Check sheet for the drawn part. Datum: minimum x, y, z corner. Units: mm. A direction names the side the tool comes from. Round coordinates to 2 decimals unless told otherwise and drop trailing zeros. Order: outer loops, then holes, each group sorted by start corner. A loop starts at its lowest first (then second) coordinate and runs counter-clockwise, first axis right, second up. Notation, with made-up numbers: (21, 32.5) -> (46, 32.5) arc R12 cw to (46, 53.5) -> close; hole circle Ø9 at (88, 28). An arc over 180 degrees is marked (long way). Answer as a JSON object with one key per item and string values. Group by question number.
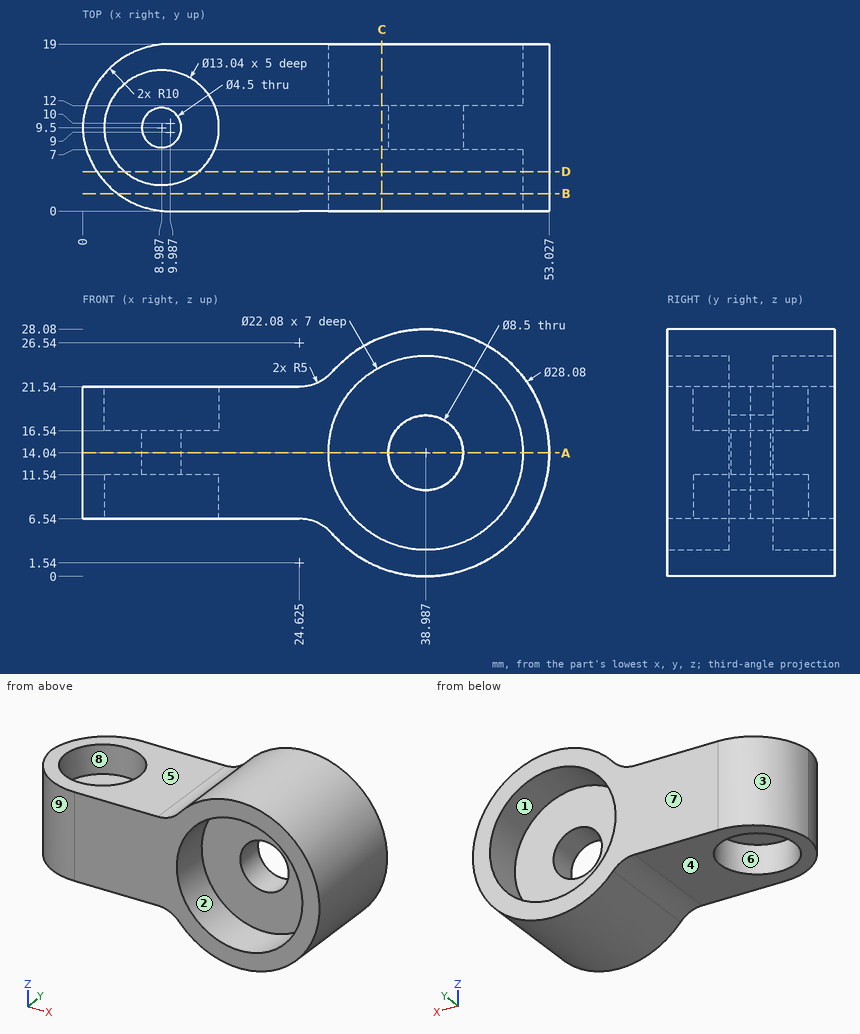
Item 1: Sectioned sample at A-A, the plane z = 14.04. Enter the section's corners in (x, y), then the cut area to 3 significant figures.
Item 2: Thickness scan on L1, parallel to X at y = 8.3, z = 14.04 (1 decimal); L2, parallel to X at y = 15.5, z = 20 (1 decimal); L3, parallel to Y at x = 29, z = 18.25. Record the ranges inside material, lowest first.
Item 3: Mould release check, pull along Y, two halves, no side actions. Record for the marked faces 6, 7, 8 and 9: pulls with the +Y half, pulls with the -Y half, needs draft (parallel to the pull), parting line crosses it, or undercut.
Item 4: Sectioned sample at D-D, the plane y = 4.5. Enter the section's corners in (x, z) (1 decimal).
Item 5: Set-up check for the marked faces 1, 2, 3, 4 and 5: record each of +Z, -Z, +X, -X, +Y, -Y from which the full face is reachable in a straight line by a thin tool's end or side.
Item 6: Depth check by flat-ended pin: pin 1 Ø8 at (x, y) = (21.5, 3) entering from -Z; pin 2 Ø5 at (x, y) = (8.99, 9.5) entering from +Z; pin 3 Ø5.5 at (x, y) = (13.5, 11.5) entering from +Z. Enter the tip coordinate at first touch or a pass-through.
Item 7: Sectioned sample at B-B, the plane y = 2. Enter the section's corners in (x, z) (1 decimal), then the cut area to 3 significant figures.
Item 8: Sectioned sample at C-C, the plane x = 34. Enter the section's corners in (y, z) (1 decimal).
Result:
{
 "1": {"outline": "(0, 9.5) arc R10 ccw to (9.99, 0) -> (27.95, 0) -> (27.95, 7) -> (34.74, 7) -> (34.74, 12) -> (27.95, 12) -> (27.95, 19) -> (9.99, 19) arc R10 ccw to start; (43.24, 7) -> (50.03, 7) -> (50.03, 0) -> (53.03, 0) -> (53.03, 19) -> (50.03, 19) -> (50.03, 12) -> (43.24, 12) -> close; hole circle Ø4.5 at (8.99, 9.5)", "area": "597 mm2"},
 "2": {"L1": "x = 0.1 to 7.1, 10.9 to 34.7, 43.2 to 53", "L2": "x = 2.4 to 6.4, 11.5 to 29.7, 48.3 to 51.7", "L3": "y = 7 to 12"},
 "3": {"face 6": "undercut", "face 7": "pulls with the +Y half", "face 8": "undercut", "face 9": "pulls with the -Y half"},
 "4": {"outline": "(1.6, 6.5) -> (4.8, 6.5) -> (4.8, 11.5) -> (13.2, 11.5) -> (13.2, 6.5) -> (24.6, 6.5) arc R5 cw to (28.4, 4.8) arc R14 ccw (long way) to (28.4, 23.3) arc R5 cw to (24.6, 21.5) -> (13.2, 21.5) -> (13.2, 16.5) -> (4.8, 16.5) -> (4.8, 21.5) -> (1.6, 21.5) -> close; hole circle Ø22.1 at (39, 14)"},
 "5": {"face 1": "+Y", "face 2": "-Y", "face 3": "+Z, -Z, -X, +Y", "face 4": "-Z, -X, +Y, -Y", "face 5": "+Z, -X, +Y, -Y"},
 "6": {"pin 1": "stops at z = 6.46", "pin 2": "stops at z = 16.54", "pin 3": "stops at z = 21.54"},
 "7": {"outline": "(4, 6.5) -> (24.6, 6.5) arc R5 cw to (28.4, 4.8) arc R14 ccw (long way) to (28.4, 23.3) arc R5 cw to (24.6, 21.5) -> (4, 21.5) -> close; hole circle Ø22.1 at (39, 14)", "area": "563 mm2"},
 "8": {"outline": "(0, 0.9) -> (19, 0.9) -> (19, 4.2) -> (12, 4.2) -> (12, 23.9) -> (19, 23.9) -> (19, 27.2) -> (0, 27.2) -> (0, 23.9) -> (7, 23.9) -> (7, 4.2) -> (0, 4.2) -> close"}
}
